```python
from build123d import *

# Parameters (mm, degrees)
F0_W     = 220
F0_H     = 380
F1_DEPTH = 120
F3_DEPTH = 220
F4_R     = 12.5
F5_DEPTH = 25


with BuildPart() as f1:
    # F0 (on Right) → F1 (new body)
    with BuildSketch(Plane.YZ):
        Rectangle(F0_W, F0_H)
    extrude(amount=-F1_DEPTH)

    # F2 (on face) → F3 (cut)
    with BuildSketch(Plane.XZ.offset(110)):
        Polygon((0, 190), (-60, 190), (0, 130), align=None)
    extrude(amount=-F3_DEPTH, mode=Mode.SUBTRACT)

    # F4 (on face) → F5 (cut)
    with BuildSketch(Plane(origin=(0, 0, -190), x_dir=(1, 0, 0), z_dir=(0, 0, -1))):
        with Locations((-60, 60)):
            Circle(F4_R)
        with Locations((-60, -60)):
            Circle(F4_R)
    extrude(amount=-F5_DEPTH, mode=Mode.SUBTRACT)


solid = f1.part
```
Geometry: final body of the model. Coordinates: model frame, mm. A direction names the side the tool comes from. Coordinates: 2 decimals unless noted, no trailing zeros. Write each loop counter-clockwise with the first axis right and the second up, starting at its lowest first coordinate (ties: lowest second). Pieces come first, ordered by that corner, then holes. Notation, with made-up numbers: M 53.5,19 L 69.5,19 A14 cw 69.5,38 Z; hole C 85,63 d11. An arc over 180 degrees is marked long. Use CSV: the item, a comma, the result in double quotes. Start each with the question number.
1. Mould query, pull axis Y, two halves, no side actions, for faces 1 (the face through (-30, -2, 160)), 2 (the face through (-59, -110, -3)), 3 (the face through (-61.627, -72.394, -177.675)). Classes: pulls with the +Y half, pulls with the -Y half, needs draft (parallel to the pull), parting line crosses it, or undercut.
2. Ray query, probe 1 along Y at (x, z) = (-60, -172); probe 2 along X at (y, z) = (-60, -171); probe 3 along Z at (x, y) = (-34, -94). Return the intervals inside material, ascending.
3. Cut plane A-A on y = -60. Return the cut outline in (x, z).
4. First-contact query: P1, Ø8, axis at y = 86, z = -53, coming from the +X side. Flat tip, straight axial feed; report the tip coordinate or a pass-through.
5. Cut plane C-C on z = 142.5. Return the cut outline in (x, y), plus the area to 4 significant figures.
6. Cut plane D-D on y = -37.5. Return the cut outline in (x, z).
7. Reachability of faces 4 (the face through (-59, 110, -3)), 5 (the face through (-61.627, 47.606, -177.675)) from +Z, -Z, +X, -X, +Y, -Y: full face, straight path, thin tool, end or side. Return the list, or none.
8. Cut plane B-B on x = -56. Return the cut outline in (y, z).
Entries:
1,face 1,"needs draft"
1,face 2,"pulls with the -Y half"
1,face 3,"undercut"
2,probe 1,"-110 to -72.5, -47.5 to 47.5, 72.5 to 110"
2,probe 2,"-120 to -72.5, -47.5 to 0"
2,probe 3,"-190 to 164"
3,outline,"M -120,-190 L -72.5,-190 L -72.5,-165 L -47.5,-165 L -47.5,-190 L 0,-190 L 0,130 L -60,190 L -120,190 Z"
4,P1,"x = 0"
5,outline,"M -120,-110 L -12.5,-110 L -12.5,110 L -120,110 Z"
5,area,"23,650 mm²"
6,outline,"M -120,-190 L 0,-190 L 0,130 L -60,190 L -120,190 Z"
7,face 4,"+Z, -Z, +X, -X, +Y"
7,face 5,"-Z"
8,outline,"M -110,-190 L -71.84,-190 L -71.84,-165 L -48.16,-165 L -48.16,-190 L 48.16,-190 L 48.16,-165 L 71.84,-165 L 71.84,-190 L 110,-190 L 110,186 L -110,186 Z"
